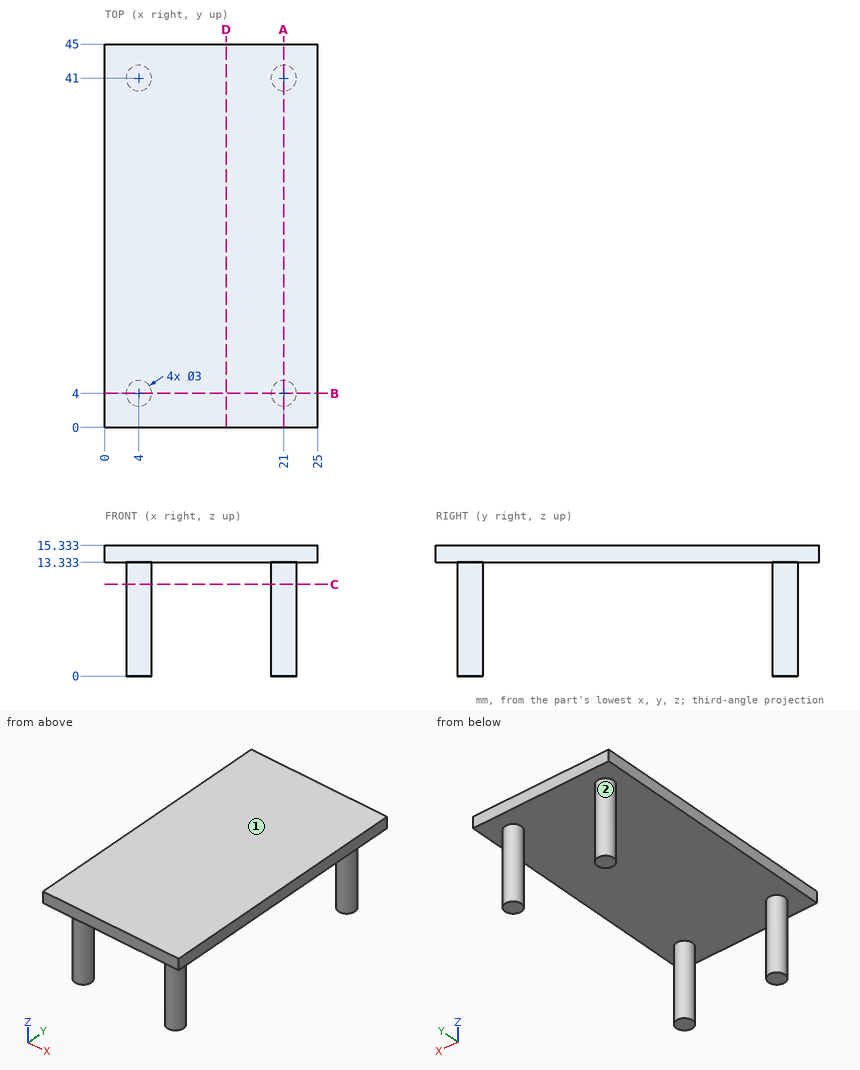
Geometry check sheet. Reference: drawing and pictorial views, mm from the part's lowest x, y, z. Coordinates: 2 decimals unless noted, no trailing zeros. Write each loop counter-clockwise with the first axis right and the second up, starting at its lowest first coordinate (ties: lowest second). Pieces come first, ordered by that corner, then holes. Notation, with made-up numbers: (55, 53) -> (103, 53) arc R7 cw to (103, 63) -> close; hole circle Ø6 at (42, 70.5). An arc over 180 degrees is marked (long way). One line per question, with ' | ' between items.
1. Cross-section at B-B on y = 4. Record the cut outline in (x, z).
Answers:
outline: (0, 13.33) -> (2.5, 13.33) -> (2.5, 0) -> (5.5, 0) -> (5.5, 13.33) -> (19.5, 13.33) -> (19.5, 0) -> (22.5, 0) -> (22.5, 13.33) -> (25, 13.33) -> (25, 15.33) -> (0, 15.33) -> close
2. Cross-section at C-C on z = 10.75. Record the cut outline in (x, y), and give its area (3 significant figures).
Answers:
outline: circle Ø3 at (4, 4); circle Ø3 at (4, 41); circle Ø3 at (21, 4); circle Ø3 at (21, 41) | area: 28.3 mm²
3. Cross-section at D-D on x = 14.25. Record the cut outline in (y, z).
Answers:
outline: (0, 13.33) -> (45, 13.33) -> (45, 15.33) -> (0, 15.33) -> close
4. Thickness scan on probe 1 along Z at (x, y) = (13.5, 5); probe 2 along Y at (x, z) = (21.5, 3.5) (1 decimal); probe 3 along Y at (x, z) = (3, 3.5). Record the ranges inside material, lowest first. Write a range as from..to.
Answers:
probe 1: z = 13.33..15.33 | probe 2: y = 2.6..5.4, 39.6..42.4 | probe 3: y = 2.88..5.12, 39.88..42.12
5. Draft check along Y on the marked faces 1 and 2. Enter one of: +Y half, -Y half, draft (parallel to the pull), parting line (faces both ways), or undercut.
Answers:
face 1: draft | face 2: undercut
6. Cross-section at A-A on x = 21. Record the cut outline in (y, z), and give its area (3 significant figures).
Answers:
outline: (0, 13.33) -> (2.5, 13.33) -> (2.5, 0) -> (5.5, 0) -> (5.5, 13.33) -> (39.5, 13.33) -> (39.5, 0) -> (42.5, 0) -> (42.5, 13.33) -> (45, 13.33) -> (45, 15.33) -> (0, 15.33) -> close | area: 170 mm²
7. Depth check by flat-ended pin: pin 1 Ø5 at (x, z) = (21, 5.5) entering from +Y. Enter the tip coordinate at first touch or a pass-through.
Answers:
pin 1: stops at y = 42.5
